The model under review builds one solid part; all positions refer to its coordinate system, in mm. A direction names the side the tool comes from. Round coordinates to 2 decimals unless told otherwise and drop trailing zeros. Write each loop counter-clockwise with the first axis right and the second up, starting at its lowest first coordinate (ties: lowest second). Pieces come first, ordered by that corner, then holes. Notation, with made-up numbers: (-5, -30.5) - (1, -30.5) arc R14 ccw to (1, -21.5) - close; hole circle Ø8 at (65.25, -13.5). An arc over 180 degrees is marked (long way). Use one line per item in the form item = value.
from build123d import *

# Parameters (mm, degrees)
SKETCH1_W           = 20
SKETCH1_H           = 20
BOSS_EXTRUDE1_DEPTH = 550
SKETCH2_R           = 5
BOSS_EXTRUDE2_DEPTH = 266.7
SKETCH3_W           = 5
SKETCH3_H           = 35
BOSS_EXTRUDE3_DEPTH = 5
LPATTERN1_COUNT     = 28
LPATTERN1_PITCH     = 20.1852


with BuildPart() as part:
    # Sketch1 → Boss-Extrude1 (new body)
    with BuildSketch(Plane.XY):
        with Locations((-10, 10)):
            Rectangle(SKETCH1_W, SKETCH1_H)
    extrude(amount=BOSS_EXTRUDE1_DEPTH)

    # Sketch2 → Boss-Extrude2 (add)
    with BuildSketch(Plane.ZY.offset(20)):
        with Locations(Location((540, 10, 0), (0, 0, 90))):
            Circle(SKETCH2_R)
    extrude(amount=BOSS_EXTRUDE2_DEPTH)

    # Sketch3 → Boss-Extrude3 (add)
    with BuildSketch(Plane.XY.offset(550)):
        with Locations((-2.5, -17.5)):
            Rectangle(SKETCH3_W, SKETCH3_H)
    boss_extrude3 = extrude(amount=-BOSS_EXTRUDE3_DEPTH)

    # LPattern1: Boss-Extrude3 ×28
    with Locations(*[(0, 0, -i * LPATTERN1_PITCH) for i in range(1, LPATTERN1_COUNT)]):
        add(boss_extrude3)


solid = part.part
(1) Machinability: for faces 4 (the cylindrical face through (-151.483, 9.349, 535.043)), 5 (the flat face through (-8, 5, 550)), which of the approach directions +Z, -Z, +X, -X, +Y, -Y give a long, thin tool a straight path to every point of the face, cutting with its end or side? Answer none if there is none.
Geometry results:
face_4 = -X
face_5 = +Z, +X, -X, +Y, -Y
(2) Add section A-A on y = 10. Write out the cut boundary in (x, z).
Geometry results:
outline = (-286.7, 535) - (-20, 535) - (-20, 0) - (0, 0) - (0, 550) - (-20, 550) - (-20, 545) - (-286.7, 545) - close
(3) Add section C-C on x = -101. Write out the cut boundary in (y, z), then the cut area to 3 significant figures.
Geometry results:
outline = circle Ø10 at (10, 540)
area = 78.5 mm2
(4) Insertion check: P1, Ø8, axis at y = -21.5, z = 473.5, coming from the -X side; P2, Ø2.5, axis at y = -20, z = 325.5, coming from the -X side; P3, Ø2, axis at y = 5.5, z = 343.5, coming from the -X side; P4, Ø3, axis at x = -192, y = 5.5, coming from the -Z side. Each pin has a flat end and moves straight along its axis. Give the tip position at first contact, or say it passes through.
Geometry results:
P1 = through
P2 = -5
P3 = -20
P4 = 536
(5) Add section D-D on y = -13.5. Count the separate pieces of the cut face and the enclosed holes in it, then the cut area to 3 significant figures.
Geometry results:
separate_pieces = 28
enclosed_holes = 0
area = 700 mm2
(6) Add section B-B on z = 540. Write out the cut boundary in (x, y).
Geometry results:
outline = (-286.7, 5) - (-20, 5) - (-20, 0) - (0, 0) - (0, 20) - (-20, 20) - (-20, 15) - (-286.7, 15) - close
(7) To check wall thickness, follow L1, parallel to X at y = 9, z = 46; L2, parallel to Y at x = -19, z = 59; L3, parallel to Z at x = -87.5, y = 9. State the ranges of each line that lie inside material, in increasing order.
Geometry results:
L1 = -20 to 0
L2 = 0 to 20
L3 = 535.1 to 544.9
(8) The part is to be moulded in two halves that separate along Z. For faces 1 (the flat face through (0, 11, 276)), 2 (the flat face through (-10, 10, 0)), 3 (the flat face through (-10, 0, 271)), say which applies: +Z half, -Z half, draft (parallel to the pull), parting line (faces both ways), or undercut.
Geometry results:
face_1 = draft
face_2 = -Z half
face_3 = undercut
